Here's how the part is built. I have some questions about the finished solid (model axes, mm). Face numbers are marked on the shaded views. Round coordinates to 2 decimals unless told otherwise and drop trailing zeros. Order: outer loops, then holes, each group sorted by start corner. A loop starts at its lowest first (then second) coordinate and runs counter-clockwise, first axis right, second up.
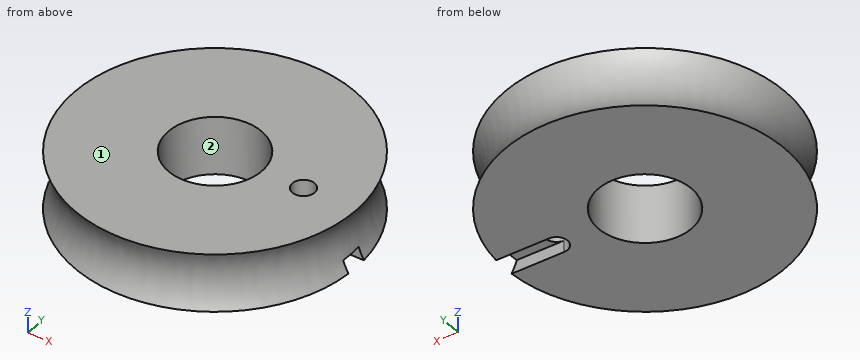
```python
from build123d import *

# Parameters (mm, degrees)
ESQUISSE2_R             = 4
ENL_V_MAT_EXTRU_1_DEPTH = 10
ESQUISSE3_R             = 0.95
ENL_V_MAT_EXTRU_2_DEPTH = 5
ESQUISSE5_W             = 5
ESQUISSE5_H             = 1.9
ENL_V_MAT_EXTRU_4_DEPTH = 1


with BuildPart() as part:
    # Esquisse1 → Révolution1 (revolve)
    with BuildSketch(Plane(origin=(0, 0, 0), x_dir=(1, 0, 0), z_dir=(0, 1, 0))):
        with BuildLine():
            Line((0, 0), (0, 5))
            Line((0, 5), (12, 5))
            ThreePointArc((12, 5), (11.330127019, 2.5), (12, 0))
            Line((12, 0), (0, 0))
        make_face()
    revolve(axis=Axis((0, 0, 0), (0, 0, -1)))

    # Esquisse2 → Enlèv. mat.-Extru.1 (cut)
    with BuildSketch(Plane(origin=(0, 0, -5), x_dir=(-1, 0, 0), z_dir=(0, 0, -1))):
        Circle(ESQUISSE2_R)
    extrude(amount=-ENL_V_MAT_EXTRU_1_DEPTH, mode=Mode.SUBTRACT)

    # Esquisse3 → Enlèv. mat.-Extru.2 (cut)
    with BuildSketch(Plane(origin=(0, 0, -5), x_dir=(-1, 0, 0), z_dir=(0, 0, -1))):
        with Locations((-7.5, 0)):
            Circle(ESQUISSE3_R)
    extrude(amount=-ENL_V_MAT_EXTRU_2_DEPTH, mode=Mode.SUBTRACT)

    # Esquisse5 → Enlèv. mat.-Extru.4 (cut)
    with BuildSketch(Plane(origin=(0, 0, -5), x_dir=(-1, 0, 0), z_dir=(0, 0, -1))):
        with Locations((-10, 0)):
            Rectangle(ESQUISSE5_W, ESQUISSE5_H)
    extrude(amount=-ENL_V_MAT_EXTRU_4_DEPTH, mode=Mode.SUBTRACT)


solid = part.part
```
1. I'm going to push flat-ended pins straight in: P1, Ø2, axis at x = -9, z = -3.5, coming from the +Y side; P2, Ø0.8, axis at x = 11, z = -4.5, coming from the -Y side; P3, Ø1.5, axis at x = 5.5, z = -1, coming from the -Y side; P4, Ø13, axis at x = 0, y = 0, coming from the +Z side. Where does each tip first touch, or does it pass through?
Evaluation:
P1: stops at y = 8.22
P2: stops at y = -5.17
P3: stops at y = -10.66
P4: stops at z = 0
2. If we section it at A-A, the plane x = 0: Write out the boundary of the cut face in (y, z), and give its area (3 significant figures).
Evaluation:
outline: (-12, -5) - (-4, -5) - (-4, 0) - (-12, 0) arc R5 cw to start; (4, -5) - (12, -5) arc R5 cw to (12, 0) - (4, 0) - close
area: 75.5 mm2
3. I need wall thicknesses on probe 1 along Z at (x, y) = (9.25, -0.75); probe 2 along Y at (x, z) = (3.5, -2.9); probe 3 along Y at (x, z) = (0, -1.5). Which ranges of each line are inside material? Lowest first, please.
Evaluation:
probe 1: z = -4 to 0
probe 2: y = -10.79 to -1.94, 1.94 to 10.79
probe 3: y = -11.43 to -4, 4 to 11.43
4. If we mould it in two halves opening along Y, with no side actions, what happens to the marked faces 1 and 2? For each: released by +Y, released by -Y, zero draft, split by the parting line, or undercut.
Evaluation:
face 1: zero draft
face 2: undercut
5. If we section it at D-D, the plane z = -3.2: Write out the boundary of the cut face in (x, y).
Evaluation:
outline: circle Ø22.76 at (0, 0); hole circle Ø8 at (0, 0); hole circle Ø1.9 at (7.5, 0)
6. If we section it at B-B, the plane y = 0: Write out the boundary of the cut face in (x, z).
Evaluation:
outline: (-12, -5) - (-4, -5) - (-4, 0) - (-12, 0) arc R5 cw to start; (4, -5) - (6.55, -5) - (6.55, 0) - (4, 0) - close; (8.45, -4) - (11.56, -4) arc R5 cw to (12, 0) - (8.45, 0) - close
7. If we section it at C-C, the plane z = -4.55: Write out the boundary of the cut face in (x, y), and give its area (3 significant figures).
Evaluation:
outline: (7.5, -0.95) arc R0.95 cw to (7.5, 0.95) - (11.73, 0.95) arc R11.77 ccw (long way) to (11.73, -0.95) - close; hole circle Ø8 at (0, 0)
area: 375 mm2
